from build123d import *

# Parameters (mm, degrees)
SKETCH_1_R          = 4
SKETCH_1_R_2        = 1.5
EXTRUDE_1_DEPTH     = 5.67
SKETCH_3_R          = 1.5
CUT_EXTRUDE_1_DEPTH = 11.96266391


with BuildPart() as part:
    # 草图1 → 凸台-拉伸1 (new body)
    with BuildSketch(Plane(origin=(0, 0, 0), x_dir=(1, 0, 0), z_dir=(0, 1, 0))):
        with Locations(Location((0, 0, 0), (0, 0, 90))):
            Circle(SKETCH_1_R)
        with Locations(Location((0, 0, 0), (0, 0, 90))):
            Circle(SKETCH_1_R_2, mode=Mode.SUBTRACT)
    extrude(amount=EXTRUDE_1_DEPTH)

    # 草图2 → 旋转1 (revolve)
    with BuildSketch(Plane.XY, mode=Mode.PRIVATE) as revolve_1_sk:
        Polygon((0, 5.67), (5.3, 5.67), (2.97, 8), (0, 8), align=None)
    revolve(revolve_1_sk.sketch.rotate(Axis((0, 5.67, 0), (0, 1, 0)), 90), axis=Axis((0, 5.67, 0), (0, 1, 0)))

    # 草图3 → 切除-拉伸1 (cut, through all)
    with BuildSketch(Plane(origin=(0, 8, 0), x_dir=(1, 0, 0), z_dir=(0, 1, 0))):
        with Locations(Location((0, 0, 0), (0, 0, 90))):
            Circle(SKETCH_3_R)
    extrude(amount=-CUT_EXTRUDE_1_DEPTH, mode=Mode.SUBTRACT)


solid = part.part
Design review of the part built by this model. Coordinates are the model's own, in mm. A direction names the side the tool comes from. Give positions to 0.01 mm unless a question says otherwise; leave off trailing zeros. Order: outer loops, then holes, each group sorted by start corner. A loop starts at its lowest first (then second) coordinate and runs counter-clockwise, first axis right, second up. Notation, with made-up numbers: (-16, 54.5) - (5, 54.5) arc R28 ccw to (5, 83.5) - close; hole circle Ø10 at (-2.5, 43.5). An arc over 180 degrees is marked (long way). Use CSV: the item, a comma, the result in double quotes. Start each with the question number.
Q1. For P1, Ø1.8, axis at x = 0, z = 0, coming from the -Y side; P2, Ø1, axis at y = 3, z = 1, coming from the +X side, all flat-tipped, find the tip position at first contact; note any pin that passes through.
Q2. Take a section at C-C (y = 6). State the section outline as (x, z) points.
Q3. Take a section at D-D (y = 7.5). State the section outline as (x, z) points.
Q4. Machinability: for faces 4 (the face through (-4, 5.67, 2)), 5 (the face through (0, 0, -2)), which of the approach directions +Z, -Z, +X, -X, +Y, -Y give a long, thin tool a straight path to every point of the face, cutting with its end or side? Answer none if there is none.
Q5. For line 1 (X direction, y = 5, z = 0); line 2 (X direction, y = 2.75, z = -1.25); line 3 (Z direction, x = 0.25, y = 6.25), list the stretches that pass through material, from the lowest coordinate up.
Q6. Take a section at B-B (x = 0). State the section outline as (y, z) points, and give its area (3 significant figures).
Q7. Take a section at A-A (z = 0). State the section outline as (x, y) points, and give its area (3 significant figures).
Q8. Draft analysis for pull direction X (two halves, no side actions). For faces 1 (the face through (1.3, 8, -1.3)), 2 (the face through (-0.45, 4.06, -1.43)), 3 (the face through (-0.926, 7.887, -2.941)), state which applies: pulls with the +X half, pulls with the -X half, needs draft (parallel to the pull), parting line crosses it, or undercut.
Calculated:
1,P1,"passes through"
1,P2,"stops at x = 3.97"
2,outline,"circle Ø9.94 at (0, 0); hole circle Ø3 at (0, 0)"
3,outline,"circle Ø6.94 at (0, 0); hole circle Ø3 at (0, 0)"
4,face 4,"-Y"
4,face 5,"+Z, -Z, +X, -X, -Y"
5,line 1,"x = -4 to -1.5, 1.5 to 4"
5,line 2,"x = -3.8 to -0.83, 0.83 to 3.8"
5,line 3,"z = -4.71 to -1.48, 1.48 to 4.71"
6,outline,"(0, -4) - (5.67, -4) - (5.67, -5.3) - (8, -2.97) - (8, -1.5) - (0, -1.5) - close; (0, 1.5) - (8, 1.5) - (8, 2.97) - (5.67, 5.3) - (5.67, 4) - (0, 4) - close"
6,area,"40.6 mm²"
7,outline,"(-5.3, 5.67) - (-4, 5.67) - (-4, 0) - (-1.5, 0) - (-1.5, 8) - (-2.97, 8) - close; (1.5, 0) - (4, 0) - (4, 5.67) - (5.3, 5.67) - (2.97, 8) - (1.5, 8) - close"
7,area,"40.6 mm²"
8,face 1,"needs draft"
8,face 2,"undercut"
8,face 3,"parting line crosses it"
